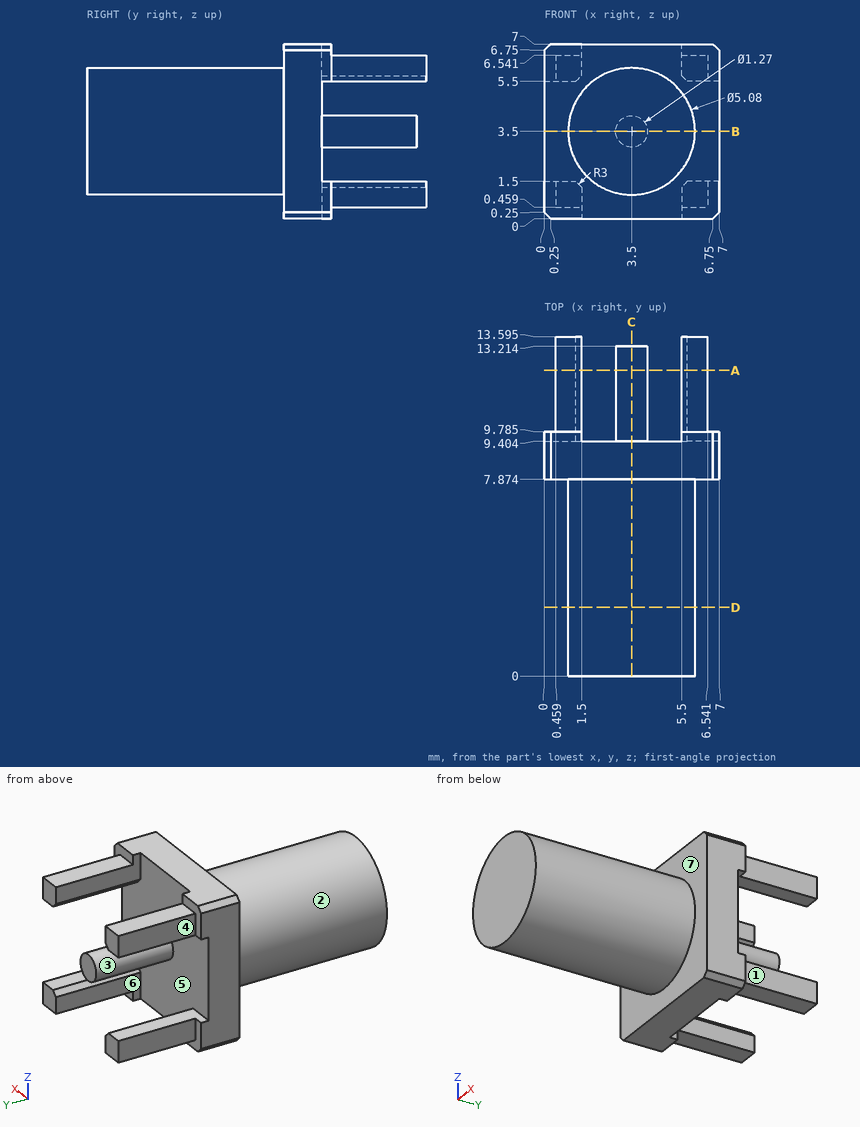
Could you check a few things on this drawing? It's one solid part, dimensions in mm from its lowest x, y, z. A direction names the side the tool comes from. Round coordinates to 2 decimals unless told otherwise and drop trailing zeros. Write each loop counter-clockwise with the first axis right and the second up, starting at its lowest first coordinate (ties: lowest second). Pieces come first, ordered by that corner, then holes. Notation, with made-up numbers: (52.25, 88) -> (84.25, 88) arc R20 cw to (84.25, 96) -> close; hole circle Ø5 at (89.5, -34.75). An arc over 180 degrees is marked (long way). One line per item, written item: value.
1) Suppose I cut it at D-D on y = 2.75. List the corners of the cut face in (x, z) for me, plus the area to 3 significant figures.
Filled sheet:
outline: circle Ø5.08 at (3.5, 3.5)
area: 20.3 mm2
2) We'd pull the mould along Y, two halves only. Please class the marked faces 5, 6 and 7: released by +Y, released by -Y, zero draft, split by the parting line, or undercut.
Filled sheet:
face 5: released by +Y
face 6: zero draft
face 7: released by -Y
3) Suppose I cut it at A-A on y = 12.25. Give the number of separate pieces and of enclosed holes in the cut face.
Filled sheet:
separate pieces: 5
enclosed holes: 0
4) I'm going to push flat-ended pins straight in: pin 1 Ø1 at (x, z) = (6.5, 4.5) entering from -Y; pin 2 Ø1 at (y, z) = (11, 6) entering from -X; pin 3 Ø1 at (y, z) = (12, 6) entering from +X. Where does each tip first touch, or does it pass through?
Filled sheet:
pin 1: stops at y = 7.87
pin 2: stops at x = 0.46
pin 3: stops at x = 6.54
5) Suppose I cut it at C-C on x = 3.5. List the corners of the cut face in (y, z) for me (1 decimal).
Filled sheet:
outline: (0, 1) -> (7.9, 1) -> (7.9, 0) -> (9.4, 0) -> (9.4, 2.9) -> (13.2, 2.9) -> (13.2, 4.1) -> (9.4, 4.1) -> (9.4, 7) -> (7.9, 7) -> (7.9, 6) -> (0, 6) -> close
6) If I drill on line 1 (Z direction, x = 0.5, y = 10.25); line 2 (Y direction, x = 3.25, z = 2.5); line 3 (Y direction, x = 0.5, z = 3.75), over which ranges is the centre line in solid material (lowest first)? Write a range as [from, to].
Filled sheet:
line 1: z = [0.46, 1.5], [5.5, 6.54]
line 2: y = [0, 9.4]
line 3: y = [7.87, 9.4]
7) Suppose I cut it at B-B on z = 3.5. List the corners of the cut face in (x, y) for me (1 decimal).
Filled sheet:
outline: (0, 7.9) -> (1, 7.9) -> (1, 0) -> (6, 0) -> (6, 7.9) -> (7, 7.9) -> (7, 9.4) -> (4.1, 9.4) -> (4.1, 13.2) -> (2.9, 13.2) -> (2.9, 9.4) -> (0, 9.4) -> close
8) For the marked faces 1, 2, 3 and 4, which set-ups out of +Z, -Z, +X, -X, +Y, -Y let a thin tool reach every point of the face, with its end or its side?
Filled sheet:
face 1: +Z, -Z, +X, +Y
face 2: -Y
face 3: +Y
face 4: +Z, -Z, -X, +Y
